CAD build for the part. Positions are in the model's coordinates, mm. A direction names the side the tool comes from. Coordinates: 2 decimals unless noted, no trailing zeros. Order: outer loops, then holes, each group sorted by start corner. A loop starts at its lowest first (then second) coordinate and runs counter-clockwise, first axis right, second up. Notation, with made-up numbers: (-6, 59) - (40, 59) arc R13 cw to (40, 70) - close; hole circle Ø5 at (-6, 47). An arc over 180 degrees is marked (long way). Return JSON: item names as keys, results as strings.
Autodesk Inventor part; units mm, degrees
ref_plane "YZ Plane" through (0, 0, 0) normal (1, 0, 0) x (0, 1, 0)
ref_plane "XZ Plane" through (0, 0, 0) normal (0, 1, 0) x (-1, 0, 0)
ref_plane "XY Plane" through (0, 0, 0) normal (0, 0, 1) x (1, 0, 0)
sketch "Sketch1" plane through (0, 0, 0) normal (0, 0, 1) x (1, 0, 0)
  circle A0 centre (0, 0) radius 2.15
  line L0 (-10, 10) -> (-2.5, 10)
  line L1 (-2.5, 10) -> (-2.5, 8.2)
  line L2 (-2.5, 8.2) -> (-6.9272, 8.2)
  line L3 (-6.9272, 8.2) -> (-2.3772, 3.65)
  line L4 (-2.3772, 3.65) -> (2.3772, 3.65)
  line L5 (2.3772, 3.65) -> (6.9272, 8.2)
  line L6 (6.9272, 8.2) -> (2.5, 8.2)
  line L7 (2.5, 8.2) -> (2.5, 10)
  line L8 (2.5, 10) -> (10, 10)
  line L9 (10, 10) -> (10, 2.5)
  line L10 (10, 2.5) -> (8.2, 2.5)
  line L11 (8.2, 2.5) -> (8.2, 6.9272)
  line L12 (8.2, 6.9272) -> (3.65, 2.3772)
  line L13 (3.65, 2.3772) -> (3.65, -2.3772)
  line L14 (3.65, -2.3772) -> (8.2, -6.9272)
  line L15 (8.2, -6.9272) -> (8.2, -2.5)
  line L16 (8.2, -2.5) -> (10, -2.5)
  line L17 (10, -2.5) -> (10, -10)
  line L18 (10, -10) -> (2.5, -10)
  line L19 (2.5, -10) -> (2.5, -8.2)
  line L20 (2.5, -8.2) -> (6.9272, -8.2)
  line L21 (6.9272, -8.2) -> (2.3772, -3.65)
  line L22 (2.3772, -3.65) -> (-2.3772, -3.65)
  line L23 (-2.3772, -3.65) -> (-6.9272, -8.2)
  line L24 (-6.9272, -8.2) -> (-2.5, -8.2)
  line L25 (-2.5, -8.2) -> (-2.5, -10)
  line L26 (-2.5, -10) -> (-10, -10)
  line L27 (-10, -10) -> (-10, -2.5)
  line L28 (-10, -2.5) -> (-8.2, -2.5)
  line L29 (-8.2, -2.5) -> (-8.2, -6.9272)
  line L30 (-8.2, -6.9272) -> (-3.65, -2.3772)
  line L31 (-3.65, -2.3772) -> (-3.65, 2.3772)
  line L32 (-3.65, 2.3772) -> (-8.2, 6.9272)
  line L33 (-8.2, 6.9272) -> (-8.2, 2.5)
  line L34 (-8.2, 2.5) -> (-10, 2.5)
  line L35 (-10, 2.5) -> (-10, 10)
  line L36 (0, 0) -> (-30.8654, 30.8654)
  line L37 (0, 0) -> (30.8654, 30.8654)
  line L38 (0, 0) -> (42.5392, 0)
  line L39 (0, 0) -> (0, 44.3419)
  dimension "d0" = 45
  dimension "d1" = 90
  dimension "Breite" = 20
  dimension "Tiefe_Schiene" = 6.35
  dimension "d2" = 1.8
  dimension "Durchmesser_Loch" = 4.3
  dimension "Wandstaerke" = 1.8
  dimension "d3" = 1.8
  dimension "Breite_Schiene" = 5
  dimension "d4" = 5
extrude "Extrusion1" add sketch "Sketch1" along normal mid plane 100 contours L38 L13 L14 L15 L16 L17 L18 L19 L20 L21 L22 L23 L24 L25 L26 L27 L28 L29 L30 L31 L32 L33 L34 L35 L36 A0 | A0 L37 L9 L10 L11 L12 L13 L38 | A0 L39 L4 L5 L6 L7 L8 L37 | L36 L0 L1 L2 L3 L4 L39 A0
fillet "Fillet1" radius 2 4 edges at (10, 10, 0) (-10, 10, 0) (10, -10, 0) (-10, -10, 0)
fillet "Fillet2" radius 0.2 8 edges at (-2.5, 8.2, 0) (2.5, 8.2, 0) (8.2, 2.5, 0) (8.2, -2.5, 0) (-2.5, -8.2, 0) (-8.2, -2.5, 0) (-8.2, 2.5, 0) (2.5, -8.2, 0)
fillet "Fillet3" radius 0.7 16 edges at (-2.5, 10, 0) (2.5, 10, 0) (10, 2.5, 0) (10, -2.5, 0) (2.5, -10, 0) (-2.5, -10, 0) (-10, -2.5, 0) (-10, 2.5, 0) (-6.9272, -8.2, 0) (-8.2, -6.9272, 0) (6.9272, -8.2, 0) (8.2, -6.9272, 0) (8.2, 6.9272, 0) (6.9272, 8.2, 0) (-6.9272, 8.2, 0) (-8.2, 6.9272, 0)
fillet "Fillet4" radius 2 8 edges at (-3.65, 2.3772, 0) (-2.3772, 3.65, 0) (2.3772, 3.65, 0) (3.65, 2.3772, 0) (3.65, -2.3772, 0) (2.3772, -3.65, 0) (-2.3772, -3.65, 0) (-3.65, -2.3772, 0)
equation "\"d2\" = Wandstaerke"
equation "\"d3\" = Wandstaerke"
equation "\"d4\" = Breite_Schiene"
properties part number "503.015.01_ITEM_20x20_100mm"
Item 1: Drop flat-ended pins along their axis: P1, Ø1.5, axis at y = 0, z = -12, coming from the -X side; P2, Ø0.7, axis at y = 9, z = 16.5, coming from the -X side; P3, Ø1.5, axis at x = 1.5, y = 5.5, coming from the -Z side; P4, Ø1, axis at x = 9, z = -6.5, coming from the +Y side. Give the stop position or say it passes through.
Findings below:
{"P1": "stops at x = -3.65", "P2": "stops at x = -9.89", "P3": "passes through", "P4": "stops at y = 9.94"}
Item 2: Which spindle directions (+Z, -Z, +X, -X, +Y, -Y) get a long thin tool onto all of the face, cutting with end or side? Do faces 1 (the cylindrical face through (9.4, -9.43, 0.7)), 2 (the flat face through (0, 3.65, -1)), 3 (the flat face through (3.65, 0, -1)), 4 (the flat face through (-4, -8.2, -1)), 5 (the cylindrical face through (-9.43, -9.4, 0.7)). Say none if no direction does.
Findings below:
{"face 1": "+Z, -Z, +X, -Y", "face 2": "+Z, -Z, +Y", "face 3": "+Z, -Z, +X", "face 4": "+Z, -Z", "face 5": "+Z, -Z, -X, -Y"}
Item 3: Wall check: L1, parallel to X at y = 0, z = 17; L2, parallel to X at y = -1.5, z = -17.5. Give the ranges that are in metal, low to high. Write a range as [from, to].
Findings below:
{"L1": "x = [-3.65, -2.15], [2.15, 3.65]", "L2": "x = [-3.65, -1.54], [1.54, 3.65]"}
Item 4: Band-saw the part on A-A, the plane y = 0. List the corners of the cut face in (x, z), then the cut area to 3 significant figures.
Findings below:
{"outline": "(-3.65, -50) - (-2.15, -50) - (-2.15, 50) - (-3.65, 50) - close; (2.15, -50) - (3.65, -50) - (3.65, 50) - (2.15, 50) - close", "area": "300 mm²"}
Item 5: Mould opens along X. For faces 6 (the flat face through (-3.65, 0, -1)), 7 (the flat face through (-0.1, 2.4, -50)), 8 (the flat face through (-5.64, -4.37, -0.7)) say: released by +X, released by -X, zero draft, split by the parting line, or undercut.
Findings below:
{"face 6": "released by -X", "face 7": "zero draft", "face 8": "undercut"}
